Autodesk Inventor part; units mm, degrees
ref_plane "YZ Plane" through (0, 0, 0) normal (1, 0, 0) x (0, 1, 0)
ref_plane "XZ Plane" through (0, 0, 0) normal (0, 1, 0) x (-1, 0, 0)
ref_plane "XY Plane" through (0, 0, 0) normal (0, 0, 1) x (1, 0, 0)
sketch "Sketch1" plane through (0, 0, 0) normal (0, 0, 1) x (1, 0, 0)
  line L0 (0, 0) -> (200, 0)
  line L1 (200, 0) -> (200, 50)
  line L2 (200, 50) -> (0, 50)
  line L3 (0, 50) -> (0, 0)
  dimension "d0" = 200
  dimension "d1" = 50
extrude "Extrusion1" add sketch "Sketch1" along normal blind 6.731
sketch "Sketch2" plane through (0, 0, 6.731) normal (0, 0, 1) x (1, 0, 0)
  line L0 (200, 50) -> (0, 50)
  line L1 (0, 50) -> (0, 0)
  line L2 (185, 15) -> (15, 15)
  line L3 (15, 15) -> (15, 35)
  line L4 (15, 35) -> (185, 35)
  line L5 (185, 35) -> (185, 15)
  circle A0 centre (15, 42.5) radius 1.588
  circle A1 centre (185, 42.5) radius 1.588
  circle A2 centre (100, 42.5) radius 1.588
  point P0 (100, 35)
  point P1 (100, 50)
  point P2 (15, 25)
  point P3 (0, 25)
  point P4 (0, 25)
  dimension "d4" = 20
  dimension "d6" = 15
  dimension "d15" = 3.176
  dimension "d18" = 50
  dimension "d23" = 7.5
extrude "Cutout" cut sketch "Sketch2" against normal up to next
sketch "Sketch3" plane through (0, 0, 6.731) normal (0, 0, 1) x (1, 0, 0)
  line L0 (200, 0) -> (200, 50)
  line L1 (0, 50) -> (0, 0)
  line L2 (0, 35) -> (6.731, 35)
  line L3 (6.731, 35) -> (6.731, 15)
  line L4 (6.731, 15) -> (0, 15)
  line L5 (0, 15) -> (0, 35)
  line L6 (200, 35) -> (193.269, 35)
  line L7 (193.269, 35) -> (193.269, 15)
  line L8 (193.269, 15) -> (200, 15)
  line L9 (200, 15) -> (200, 35)
  point P0 (193.269, 25)
  point P1 (200, 25)
  dimension "d9" = 20
  dimension "d10" = 6.731
extrude "Tabs Neg" cut sketch "Sketch3" against normal up to next
sketch "Sketch4" plane through (0, 0, 6.731) normal (0, 0, 1) x (1, 0, 0)
  line L0 (6.731, 35) -> (6.731, 15)
  line L1 (6.731, 15) -> (0, 15)
  line L2 (0, 0) -> (200, 0)
  line L3 (90, 0) -> (110, 0)
  line L4 (110, 0) -> (110, -6.731)
  line L5 (110, -6.731) -> (90, -6.731)
  line L6 (90, -6.731) -> (90, 0)
  line L7 (200, 50) -> (0, 50)
  line L8 (90, 50) -> (110, 50)
  line L9 (110, 50) -> (110, 56.731)
  line L10 (110, 56.731) -> (90, 56.731)
  line L11 (90, 56.731) -> (90, 50)
  point P0 (100, -6.731)
  point P1 (100, 0)
extrude "Tabs Pos" add sketch "Sketch4" against normal blind 6.731
equation "\"d2\" = THICKB"
equation "\"d7\" = THICKB"
equation "\"d10\" = THICKB"
equation "\"d11\" = THICKB"
equation "\"d13\" = THICKB"
equation "\"THICKA\" = 3.175"
equation "\"THICKB\" = 6.731"
equation "\"THICKC\" = 12.7"
equation "\"THICKPLY\" = 5"
equation "\"MAGDIA\" = 9.5"
equation "\"BALLDIA\" = 12"
properties part number "Controller_Back"
Part model, mm, in its own coordinate system. A direction names the side the tool comes from. Give positions to 0.01 mm unless a question says otherwise; leave off trailing zeros. Order: outer loops, then holes, each group sorted by start corner. A loop starts at its lowest first (then second) coordinate and runs counter-clockwise, first axis right, second up. Notation, with made-up numbers: M -4,-15.75 L 30,-15.75 A34 cw 30,23.25 Z; hole C 53,32.25 d11. An arc over 180 degrees is marked long. Use a Markdown table: item, result. Add a question column.
(1) Probe line 1 along X through (y, z) = (19.5, 4.75); line 2 along Y through (x, z) = (36.5, 6); line 3 along Y through (x, z) = (108, 2.5). List the from-to ranges inside material, lowest first. Write a range as [from, to].
(2) Mould opens along X. For faces 1 (the face through (110, -3, 3)), 2 (the face through (3, 35, 3)), 3 (the face through (185, 25, 3)) say: +X half, -X half, draft (parallel to the pull), parting line (faces both ways), or undercut.
(3) 3-axis set-ups, long thin cutter, end or side, ignore diameter. For faces 4 (the face through (156, 50, 3)), 5 (the face through (15, 25, 3)), 6 (the face through (154, 0, 3)), 7 (the face through (90, -3, 3)), 8 (the face through (3, 15, 3)): which of +Z, -Z, +X, -X, +Y, -Y reach the whole face in a straight line?
(4) Saw through at B-B, the plane z = 5.5. Give the cut face in (x, y).
(5) Saw through at A-A, the plane y = 30.5. Give the cut face in (x, z), and give its area (3 significant figures).
(6) Drop flat-ended pins along their axis: P1, Ø3.5, axis at x = 4.5, z = 2, coming from the -Y side; P2, Ø6, axis at x = 76, y = 30.5, coming from the +Z side; P3, Ø2, axis at y = -3, z = 2, coming from the -X side; P4, Ø1, axis at y = 25, z = 1, coming from the +X side. Give the stop position or say it passes through.
Answer key:
| question | item | result |
|---|---|---|
| 1 | line 1 | [6.73, 15], [185, 193.27] |
| 1 | line 2 | [0, 15], [35, 50] |
| 1 | line 3 | [-6.73, 15], [35, 56.73] |
| 2 | face 1 | +X half |
| 2 | face 2 | draft |
| 2 | face 3 | undercut |
| 3 | face 4 | +Z, -Z, +X, +Y |
| 3 | face 5 | +Z, -Z |
| 3 | face 6 | +Z, -Z, +X, -Y |
| 3 | face 7 | +Z, -Z, -X, -Y |
| 3 | face 8 | +Z, -Z, -X |
| 4 | outline | M 0,0 L 90,0 L 90,-6.73 L 110,-6.73 L 110,0 L 200,0 L 200,15 L 193.27,15 L 193.27,35 L 200,35 L 200,50 L 110,50 L 110,56.73 L 90,56.73 L 90,50 L 0,50 L 0,35 L 6.73,35 L 6.73,15 L 0,15 Z; hole C 15,42.5 d3.18; hole M 15,15 L 185,15 L 185,35 L 15,35 Z; hole C 100,42.5 d3.18; hole C 185,42.5 d3.18 |
| 5 | outline | M 6.73,0 L 15,0 L 15,6.73 L 6.73,6.73 Z; M 185,0 L 193.27,0 L 193.27,6.73 L 185,6.73 Z |
| 5 | area | 111 mm^2 |
| 6 | P1 | y = 0 |
| 6 | P2 | through |
| 6 | P3 | x = 90 |
| 6 | P4 | x = 193.27 |
